Verification items for the finished model (mm, model axes). Face numbers are marked on the shaded views. A direction names the side the tool comes from. Coordinates: 2 decimals unless noted, no trailing zeros. Order: outer loops, then holes, each group sorted by start corner. A loop starts at its lowest first (then second) coordinate and runs counter-clockwise, first axis right, second up. Notation, with made-up numbers: M 3,12.5 L 38,12.5 A24 cw 38,38.5 Z; hole C 56,73.5 d9. An arc over 180 degrees is marked long. Return JSON: item names as keys, results as strings. Group by question number.
Q1. Section check A-A, the plane x = 40. Enter the section's corners in (y, z).
Q2. Go/stop test with flat-tipped pins: pin 1 Ø2 at (x, z) = (33, 3.5) entering from -Y; pin 2 Ø7 at (x, y) = (51, 5.5) entering from +Z; pin 3 Ø4 at (x, y) = (30.5, 8) entering from +Z. Record where each tip stops, or that it passes through.
Q3. Section check C-C, the plane x = 29. Enter the section's corners in (y, z).
Q4. Thickness scan on probe 1 along Y at (x, z) = (36.5, 4.4); probe 2 along Y at (x, z) = (40, 2.45); probe 3 along X at (y, z) = (-9, 4.65). Record the ranges inside material, lowest first.
Q5. Section check B-B, the plane y = 0. Enter the section's corners in (x, z).
Q6. Access from +Z, -Z, +X, -X, +Y, -Y to the whole of each face (thin tool, end or side, straight path). Record for the marked faces 1 and 2.
Q7. Section check D-D, the plane z = 0.85. Enter the section's corners in (x, y).
Q8. Mould release check, pull along X, two halves, no side actions. Record for the marked faces 3, 4 and 5: pulls with the +X half, pulls with the -X half, needs draft (parallel to the pull), parting line crosses it, or undercut.
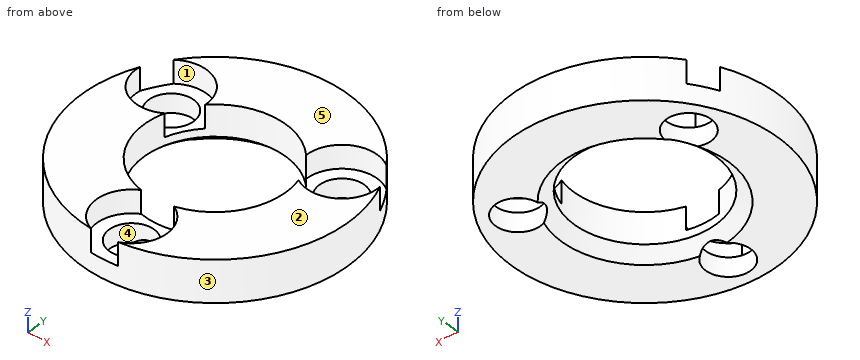
from build123d import *

# Parameters (mm, degrees)
SKETCH005_R         = 4.25
PAD005_DEPTH        = 2.75
CYLINDER_R          = 8.5
CYLINDER_DEPTH      = 11
SKETCH003_R         = 16
SKETCH003_R_2       = 2.7
PAD003_DEPTH        = 5
CUT_PLACEMENT_ANGLE = 180


with BuildPart() as pad009:
    # Sketch005 → Pad005 (new body)
    with BuildSketch(Plane(origin=(40, 0, 0), x_dir=(1, 0, 0), z_dir=(0, 0, 1))):
        with Locations((0, 12)):
            Circle(SKETCH005_R)
        with Locations((-10.392315, -5.999983)):
            Circle(SKETCH005_R)
        with Locations((10.392315, -5.999983)):
            Circle(SKETCH005_R)
    extrude(amount=PAD005_DEPTH)


with BuildPart() as cylindre:
    # Cylinder → Cylinder (new body)
    with BuildSketch(Plane(origin=(40, 0, 0), x_dir=(1, 0, 0), z_dir=(0, 0, 1))):
        Circle(CYLINDER_R)
    extrude(amount=CYLINDER_DEPTH)


with BuildPart() as fusion:
    # Cone → Cone (revolve)
    with BuildSketch(Plane(origin=(40, 0, 2), x_dir=(1, 0, 0), z_dir=(0, -1, 0))):
        Polygon((0, 0), (6.5, 0), (10, 3), (0, 3), align=None)
    revolve(axis=Axis((40, 0, 2), (0, 0, 1)))

    # Fusion: union Cylindre
    add(cylindre.part)


with BuildPart() as wheel:
    # Sketch003 → Pad003 (new body)
    with BuildSketch(Plane(origin=(40, 0, 0), x_dir=(1, 0, 0), z_dir=(0, 0, 1))):
        Circle(SKETCH003_R)
        with Locations((0, 12)):
            Circle(SKETCH003_R_2, mode=Mode.SUBTRACT)
        with Locations((-10.392315, -5.999983)):
            Circle(SKETCH003_R_2, mode=Mode.SUBTRACT)
        with Locations((10.392315, -5.999983)):
            Circle(SKETCH003_R_2, mode=Mode.SUBTRACT)
    extrude(amount=PAD003_DEPTH)

    # Cut002: cut Fusion
    add(fusion.part, mode=Mode.SUBTRACT)

    # Cut: cut Pad009
    add(pad009.part, mode=Mode.SUBTRACT)


with BuildPart() as wheel_1:
    # Cut placement: moved
    add(wheel.part.moved(Location((0, 0, 5))).rotate(Axis((0, 0, 5), (1, 0, 0)), CUT_PLACEMENT_ANGLE))


solid = wheel_1.part
Numbers:
{
 "1": {"outline": "M -16,0 L -14.7,0 L -14.7,2.25 L -16,2.25 Z; M -9.3,0.6 L -8.5,1.29 L -8.5,2.25 L -9.3,2.25 Z; M 8.5,1.29 L 10,0 L 16,0 L 16,5 L 8.5,5 Z"},
 "2": {"pin 1": "stops at y = -14.83", "pin 2": "stops at z = 5", "pin 3": "stops at z = 2.25"},
 "3": {"outline": "M -11.62,0 L 3.37,0 L 3.37,2.25 L 1.79,2.25 L 1.79,5 L -11.62,5 Z; M 8.63,0 L 11.62,0 L 11.62,5 L 10.21,5 L 10.21,2.25 L 8.63,2.25 Z"},
 "4": {"probe 1": "y = -15.61 to -14.41, -9.59 to -7.75, 7.75 to 15.61", "probe 2": "y = 8.5 to 16", "probe 3": "x = 26.77 to 36.99, 43.01 to 53.23"},
 "5": {"outline": "M 24,0 L 30,0 L 31.5,1.29 L 31.5,5 L 24,5 Z; M 48.5,1.29 L 50,0 L 56,0 L 56,5 L 48.5,5 Z"},
 "6": {"face 1": "+Z", "face 2": "+Z, +X, -X, +Y, -Y"},
 "7": {"outline": "C 40,0 d32; hole C 29.61,6 d5.4; hole C 40,0 d18.02; hole C 40,-12 d5.4; hole C 50.39,6 d5.4"},
 "8": {"face 3": "parting line crosses it", "face 4": "undercut", "face 5": "needs draft"}
}
